from build123d import *

# Parameters (mm, degrees)
SKETCH1_R           = 1.75
SKETCH1_R_2         = 1.625
SKETCH1_R_3         = 1.74995
BOSS_EXTRUDE1_DEPTH = 6.35
SKETCH2_R           = 1.74995
CUT_EXTRUDE1_DEPTH  = 122.309718695


with BuildPart() as part:
    # Sketch1 → Boss-Extrude1 (new body)
    with BuildSketch(Plane(origin=(0, 0, 0), x_dir=(1, 0, 0), z_dir=(0, 1, 0))):
        Polygon((22.35631132, -22.09368868), (22.35631132, 22.35631132), (0.13131132, 22.35631132), (-42.824896411, 96.75864561), (-72.89368868, 79.3984203), (-22.09368868, -8.589760725), (-22.09368868, -22.09368868), align=None)
        with Locations(Location((-17.829200922, -17.829200922, 0), (0, 0, 270))):
            Circle(SKETCH1_R, mode=Mode.SUBTRACT)
        with Locations(Location((0.13131132, 0.13131132, 0), (0, 0, 270))):
            Circle(SKETCH1_R_2, mode=Mode.SUBTRACT)
        with Locations(Location((18.091823562, 18.091823562, 0), (0, 0, 270))):
            Circle(SKETCH1_R_2, mode=Mode.SUBTRACT)
        with Locations(Location((18.091823562, -17.829200922, 0), (0, 0, 270))):
            Circle(SKETCH1_R_2, mode=Mode.SUBTRACT)
        with Locations(Location((-17.829200922, 18.091823562, 0), (0, 0, 270))):
            Circle(SKETCH1_R_2, mode=Mode.SUBTRACT)
        with Locations(Location((-17.723762663, 38.544433004, 0), (0, 0, 270))):
            Circle(SKETCH1_R_3, mode=Mode.SUBTRACT)
        with Locations(Location((-34.76828868, 28.70377132, 0), (0, 0, 270))):
            Circle(SKETCH1_R_3, mode=Mode.SUBTRACT)
    extrude(amount=BOSS_EXTRUDE1_DEPTH)

    # Sketch2 → Cut-Extrude1 (cut, through all)
    with BuildSketch(Plane.XZ):
        with BuildLine():
            ThreePointArc((-49.268883494, -83.359508021), (-50.810803794, -83.156510362), (-52.044647115, -84.103271641))
            Line((-52.044647115, -84.103271641), (-50.284883494, -85.119271641))
            Line((-50.284883494, -85.119271641), (-49.268883494, -83.359508021))
        make_face()
        with BuildLine():
            Line((-50.284883494, -85.119271641), (-52.044647115, -84.103271641))
            ThreePointArc((-52.044647115, -84.103271641), (-50.810803794, -87.08203292), (-48.252883494, -85.119271641))
            ThreePointArc((-48.252883494, -85.119271641), (-48.525119874, -84.103271641), (-49.268883494, -83.359508021))
            Line((-49.268883494, -83.359508021), (-50.284883494, -85.119271641))
        make_face()
        with BuildLine():
            Line((-57.323937976, -81.055271641), (-59.083701597, -80.039271641))
            Line((-59.083701597, -80.039271641), (-58.067701597, -78.279508021))
            ThreePointArc((-58.067701597, -78.279508021), (-61.046462876, -80.565191941), (-57.323937976, -81.055271641))
        make_face()
        with BuildLine():
            Line((-58.067701597, -78.279508021), (-59.083701597, -80.039271641))
            Line((-59.083701597, -80.039271641), (-57.323937976, -81.055271641))
            ThreePointArc((-57.323937976, -81.055271641), (-57.120940318, -80.565191941), (-57.051701597, -80.039271641))
            ThreePointArc((-57.051701597, -80.039271641), (-57.323937976, -79.023271641), (-58.067701597, -78.279508021))
        make_face()
        with BuildLine():
            ThreePointArc((-27.914647115, -42.308885654), (-28.117644773, -43.850805954), (-27.170883494, -45.084649275))
            Line((-27.170883494, -45.084649275), (-26.154883494, -43.324885654))
            Line((-26.154883494, -43.324885654), (-27.914647115, -42.308885654))
        make_face()
        with BuildLine():
            Line((-26.154883494, -43.324885654), (-27.170883494, -45.084649275))
            ThreePointArc((-27.170883494, -45.084649275), (-25.138883494, -45.084649275), (-24.122883494, -43.324885654))
            ThreePointArc((-24.122883494, -43.324885654), (-25.628963195, -41.362124375), (-27.914647115, -42.308885654))
            Line((-27.914647115, -42.308885654), (-26.154883494, -43.324885654))
        make_face()
        with BuildLine():
            ThreePointArc((-32.921701597, -38.244885654), (-35.969701597, -36.485122034), (-35.969701597, -40.004649275))
            Line((-35.969701597, -40.004649275), (-34.953701597, -38.244885654))
            Line((-34.953701597, -38.244885654), (-33.193937976, -39.260885654))
            ThreePointArc((-33.193937976, -39.260885654), (-32.990940318, -38.770805954), (-32.921701597, -38.244885654))
        make_face()
        with BuildLine():
            Line((-34.953701597, -38.244885654), (-35.969701597, -40.004649275))
            ThreePointArc((-35.969701597, -40.004649275), (-34.427781297, -40.207646933), (-33.193937976, -39.260885654))
            Line((-33.193937976, -39.260885654), (-34.953701597, -38.244885654))
        make_face()
        with Locations(Location((-17.723762663, -38.544433004, 0), (0, 0, 90))):
            Circle(SKETCH2_R)
        Polygon((-22.145592633, -48.57259018), (-43.735592633, -85.967567115), (-63.092992458, -74.791567115), (-41.502992458, -37.39659018), align=None)
    extrude(amount=-CUT_EXTRUDE1_DEPTH, mode=Mode.SUBTRACT)


solid = part.part
Source: CAD feature listing. Evaluate the final solid. Frame: model axes, mm. A direction names the side the tool comes from. Give positions to 0.01 mm unless a question says otherwise; leave off trailing zeros. Write each loop counter-clockwise with the first axis right and the second up, starting at its lowest first coordinate (ties: lowest second). Pieces come first, ordered by that corner, then holes. Notation, with made-up numbers: M 62,72 L 113,72 A22 cw 113,102 Z; hole C -31.75,84 d6. An arc over 180 degrees is marked long. Answer as a JSON object with one key per item and string values.
Q1. Ray query, line 1 along Z through (x, y) = (-33.5, 3.5); line 2 along Z through (x, y) = (-45, 0.5); line 3 along X through (y, z) = (0.5, -64.5). Return the intervals inside material, ascending.
Geometry check:
{"line 1": "z = -80.61 to -68.24, -42.02 to -39.66, -36.83 to -29.91, -27.5 to -11.17", "line 2": "z = -95.5 to -85.24, -43.45 to -31.09", "line 3": "x = -64.29 to -57.15, -31.34 to -24.2"}
Q2. Access query for faces 5 (the face through (11, 3, -22.356)), 6 (the face through (-18, 0, -20)), 7 (the face through (-52.45, 3.13, -56.36)). Directions: +Z, -Z, +X, -X, +Y, -Y. A direction counts if a zero-diameter tool reaches every point of the face in a straight line with its end or side. Return the directions, or none.
Geometry check:
{"face 5": "-Z, +X, +Y, -Y", "face 6": "+Z, -Z, +X, -X, -Y", "face 7": "+Y, -Y"}
Q3. Mould query, pull axis Z, two halves, no side actions, for faces 1 (the face through (0, 3, 22.094)), 2 (the face through (-32.79, 3.13, -67.01)), 3 (the face through (-18, 6.35, -20)), 4 (the face through (-21.05, 3.13, -59.04)). Classes: +Z half, -Z half, draft (parallel to the pull), parting line (faces both ways), or undercut.
Geometry check:
{"face 1": "+Z half", "face 2": "undercut", "face 3": "draft", "face 4": "-Z half"}
Q4. Contact query for flat-ended pins moving along their axis: P1, Ø1.5, axis at x = -24, y = 1, coming from the -Z side; P2, Ø2.5, axis at x = 0.13, z = -0.13, coming from the -Y side; P3, Ø3, axis at y = 2.5, z = -56, coming from the +X side; P4, Ø1.9, axis at y = 1.5, z = 17.5, coming from the -X side. Output: stop coordinate, or through.
Geometry check:
{"P1": "stops at z = -65.45", "P2": "passes through", "P3": "stops at x = -18.43", "P4": "stops at x = -22.09"}
Q5. Cut plane A-A, the plane x = -31. Return the cut outline in (y, z), then the cut area to 3 significant figures.
Geometry check:
{"outline": "M 0,-76.28 L 6.35,-76.28 L 6.35,-63.91 L 0,-63.91 Z; M 0,-43.46 L 6.35,-43.46 L 6.35,-6.84 L 0,-6.84 Z", "area": "311 mm^2"}
Q6. Cut plane B-B, the plane z = -55. Return the cut outline in (x, y), then the cut area to 3 significant figures.
Geometry check:
{"outline": "M -58.81,0 L -51.67,0 L -51.67,6.35 L -58.81,6.35 Z; M -25.86,0 L -18.72,0 L -18.72,6.35 L -25.86,6.35 Z", "area": "90.7 mm^2"}
Q7. Cut plane C-C, the plane z = -18. Return the cut outline in (x, y), then the cut area to 3 significant figures.
Geometry check:
{"outline": "M -37.45,0 L -19.45,0 L -19.45,6.35 L -37.45,6.35 Z; M -16.21,0 L 16.47,0 L 16.47,6.35 L -16.21,6.35 Z; M 19.71,0 L 22.36,0 L 22.36,6.35 L 19.71,6.35 Z", "area": "339 mm^2"}
Q8. Cut plane D-D, the plane y = 5.25. Count the separate pieces of the cut face and the enclosed holes in it, then the cut area to 3 significant figures.
Geometry check:
{"separate pieces": "1", "enclosed holes": "12", "area": "3,810 mm^2"}
